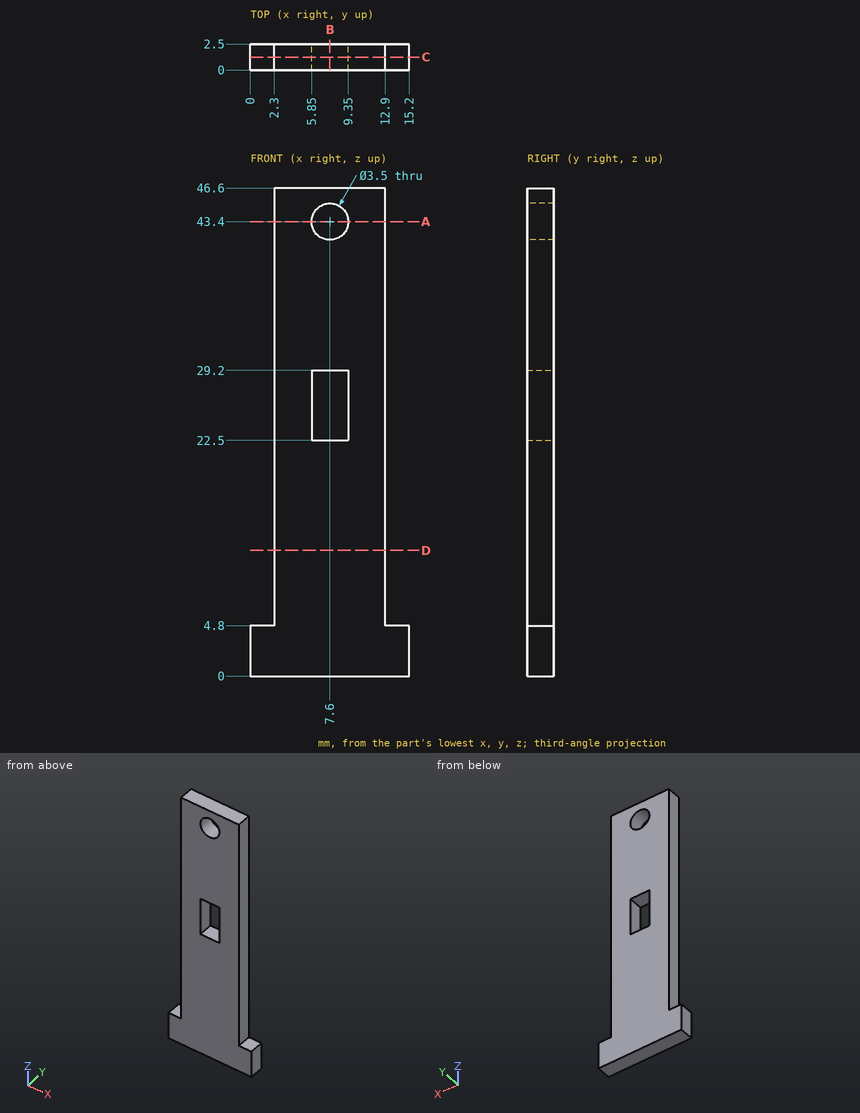
Print and shaded views of the part. All mm, measured from the part's lowest x, y and z. Give positions to 0.01 mm unless a question says otherwise; leave off trailing zeros. Loops run counter-clockwise (first coordinate to the right, second up) from the corner with the lowest first, then second, coordinate; pieces in that order, holes last. Notation, with made-up numbers: (-39.75, 88.5) - (-22.75, 88.5) arc R15 ccw to (-22.75, 101.5) - close; hole circle Ø11 at (50, -10.5). An arc over 180 degrees is marked (long way). Use a Markdown table: item, result.
(1) Band-saw the part on D-D (z = 12). Give the cut face in (x, y).
Taken from the geometry:
| item | result |
|---|---|
| outline | (2.3, 0) - (12.9, 0) - (12.9, 2.5) - (2.3, 2.5) - close |
(2) Band-saw the part on C-C (y = 1.25). Give the cut face in (x, z), and give its area (3 significant figures).
Taken from the geometry:
| item | result |
|---|---|
| outline | (0, 0) - (15.2, 0) - (15.2, 4.8) - (12.9, 4.8) - (12.9, 46.6) - (2.3, 46.6) - (2.3, 4.8) - (0, 4.8) - close; hole (5.85, 22.5) - (9.35, 22.5) - (9.35, 29.2) - (5.85, 29.2) - close; hole circle Ø3.5 at (7.6, 43.4) |
| area | 483 mm2 |
(3) Wall check: line 1 along Z through (x, y) = (7.6, 1.2); line 2 along X through (y, z) = (1.7, 43.4). Give the ranges that are in metal, low to high.
Taken from the geometry:
| item | result |
|---|---|
| line 1 | 0 to 22.5, 29.2 to 41.65, 45.15 to 46.6 |
| line 2 | 2.3 to 5.85, 9.35 to 12.9 |
(4) Band-saw the part on B-B (x = 7.6). Give the cut face in (y, z), and give its area (3 significant figures).
Taken from the geometry:
| item | result |
|---|---|
| outline | (0, 0) - (2.5, 0) - (2.5, 22.5) - (0, 22.5) - close; (0, 29.2) - (2.5, 29.2) - (2.5, 41.65) - (0, 41.65) - close; (0, 45.15) - (2.5, 45.15) - (2.5, 46.6) - (0, 46.6) - close |
| area | 91.0 mm2 |
(5) Drop flat-ended pins along their axis: pin 1 Ø1 at (x, z) = (2, 24) entering from -Y; pin 2 Ø0.8 at (y, z) = (1.5, 18) entering from -X; pin 3 Ø1.2 at (x, y) = (1.5, 1.5) entering from +Z. Give the stop position or say it passes through.
Taken from the geometry:
| item | result |
|---|---|
| pin 1 | y = 0 |
| pin 2 | x = 2.3 |
| pin 3 | z = 4.8 |
(6) Band-saw the part on A-A (z = 43.4). Give the cut face in (x, y), and give its area (4 significant figures).
Taken from the geometry:
| item | result |
|---|---|
| outline | (2.3, 0) - (5.85, 0) - (5.85, 2.5) - (2.3, 2.5) - close; (9.35, 0) - (12.9, 0) - (12.9, 2.5) - (9.35, 2.5) - close |
| area | 17.75 mm2 |
